Study the drawing (mm; zero at the part's minimum x, y, z) and answer. A direction names the side the tool comes from. Coordinates: 2 decimals unless noted, no trailing zeros. Loops run counter-clockwise (first coordinate to the right, second up) from the corner with the lowest first, then second, coordinate; pieces in that order, holes last. Notation, with made-up numbers: (44.25, 26) -> (68.25, 26) arc R5 cw to (68.25, 35) -> close; hole circle Ø3 at (63, 43). An arc over 180 degrees is marked (long way). One line per question, with ' | ' between items.
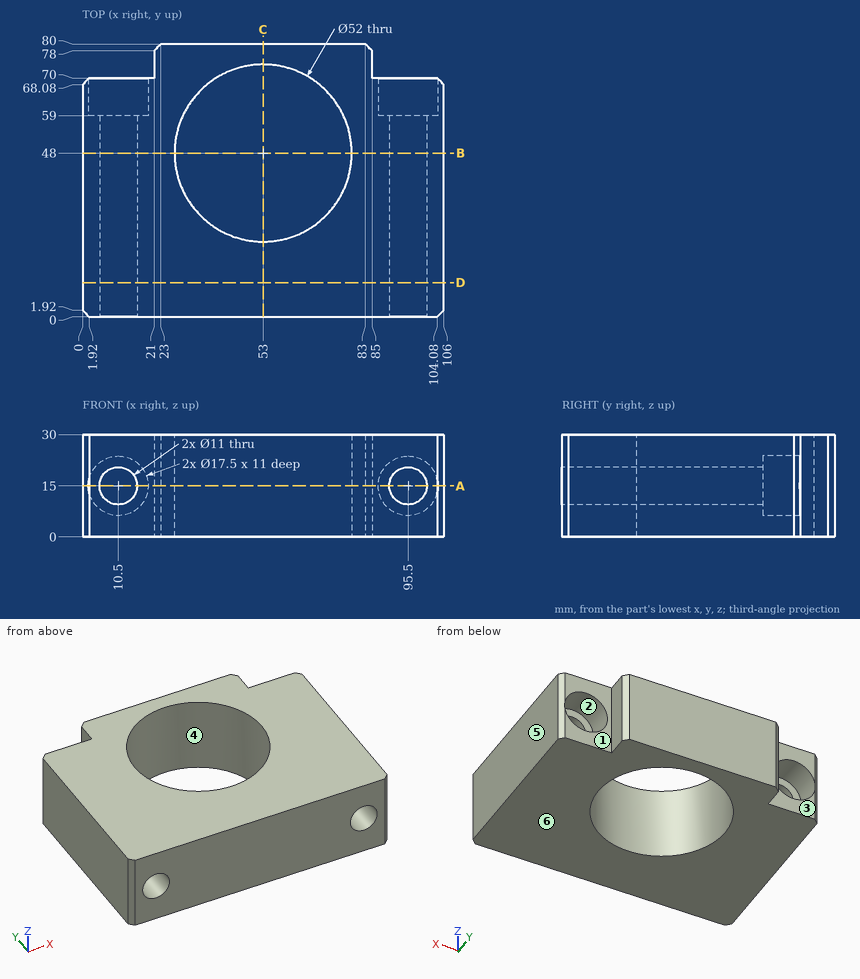
1) For the marked faces 1, 2 and 3, determine the directions among +Z, -Z, +X, -X, +Y, -Y from which every point of the face is accessible in a straight line to the end or side of a thin tool.
Check values:
face 1: +Z, -Z, +X, +Y | face 2: +Y | face 3: +Z, -Z, -X, +Y
2) Find section B-B (y = 48). Write down the section's boundary in (x, z), plus the area to 3 significant figures.
Check values:
outline: (0, 0) -> (27, 0) -> (27, 30) -> (0, 30) -> close; (79, 0) -> (106, 0) -> (106, 30) -> (79, 30) -> close; hole circle Ø11 at (10.5, 15); hole circle Ø11 at (95.5, 15) | area: 1,430 mm^2
3) Find the intervals of material crossed by line 1 along Y through (x, z) = (53, 6.5); line 2 along X through (y, z) = (67.5, 14.5); line 3 along Z through (x, y) = (95, 64), in increasing order.
Check values:
line 1: y = 0 to 22, 74 to 80 | line 2: x = 0 to 1.76, 19.24 to 35.8, 70.2 to 86.76, 104.24 to 106 | line 3: z = 0 to 6.26, 23.74 to 30
4) Find section A-A (z = 15). State how many separate pieces and enclosed holes the cut face has, plus the area to 3 significant figures.
Check values:
separate pieces: 3 | enclosed holes: 1 | area: 4,240 mm^2
5) The mould has two halves that part along X. Classify the marked faces 4, 5 and 6: released by +X, released by -X, zero draft, split by the parting line, or undercut.
Check values:
face 4: undercut | face 5: released by +X | face 6: zero draft
6) Flat-ended cylindrical pins translate along their axes: pin 1 (9 mm diameter, centred on x = 10.5, z = 15, fed in from +Y); pin 2 (15.5 mm diameter, centred on x = 10.5, z = 15, fed in from -Y); pin 3 (14 mm diameter, centred on x = 95.5, z = 15, fed in from +Y); pin 4 (3 mm diameter, centred on y = 72, z = 14.5, fed in from -X). Find the tip coordinate at first contact, or state that the pin passes through.
Check values:
pin 1: passes through | pin 2: stops at y = 0 | pin 3: stops at y = 59 | pin 4: stops at x = 21
7) Find section C-C (x = 53). Write down the section's boundary in (y, z), plus the area to 3 significant figures.
Check values:
outline: (0, 0) -> (22, 0) -> (22, 30) -> (0, 30) -> close; (74, 0) -> (80, 0) -> (80, 30) -> (74, 30) -> close | area: 840 mm^2
8) Find section D-D (y = 10). Write down the section's boundary in (x, z).
Check values:
outline: (0, 0) -> (106, 0) -> (106, 30) -> (0, 30) -> close; hole circle Ø11 at (10.5, 15); hole circle Ø11 at (95.5, 15)
